Source: CAD feature listing. Evaluate the final solid. Frame: model axes, mm. Round coordinates to 2 decimals unless told otherwise and drop trailing zeros. Order: outer loops, then holes, each group sorted by start corner. A loop starts at its lowest first (then second) coordinate and runs counter-clockwise, first axis right, second up. Notation, with made-up numbers: (-33, 56) - (-21, 56) arc R27 cw to (-21, 95) - close; hole circle Ø2 at (61.5, 56.5). An arc over 180 degrees is marked (long way). Use one line per item in the form item = value. Start each with the question number.
Q1. Cut plane C-C, the plane z = 1.45. Give the number of separate pieces and of enclosed holes in the cut face, and give its area (3 significant figures).
Q2. Cut plane B-B, the plane x = 21. Return the cut outline in (y, z), and give its area (3 significant figures).
Q3. Ray query, line 1 (X direction, y = 41, z = 0.35); line 2 (Y direction, x = 22, z = 0.55); line 3 (Y direction, x = 17, z = 2.55). Return the intervals inside material, ascending. Write a range as [from, to].
Q4. Draft query along X for faces 1 (the flat face through (80.008, 41, 1)), 2 (the flat face through (33, 43, 0)), 3 (the flat face through (59.008, 67, 2)). Return one class per face: released by +X, released by -X, zero draft, split by the parting line, or undercut.
Q5. Cut plane A-A, the plane y = 92.5. Return the cut outline in (x, z), and give its area (3 significant figures).
from build123d import *

# Parameters (mm, degrees)
ESQUISSE1_W             = 120
ESQUISSE1_H             = 140
BOSS_EXTRU_1_DEPTH      = 3
ESQUISSE3_R             = 5
ESQUISSE3_W             = 3
ESQUISSE3_H             = 10
ENL_V_MAT_EXTRU_1_DEPTH = 138.692369665


with BuildPart() as part:
    # Esquisse1 → Boss.-Extru.1 (new body)
    with BuildSketch(Plane.XY):
        with Locations((20.007954742, 42.021943574)):
            Rectangle(ESQUISSE1_W, ESQUISSE1_H)
    extrude(amount=BOSS_EXTRU_1_DEPTH)

    # Esquisse3 → Enlèv. mat.-Extru.1 (cut, through all)
    with BuildSketch(Plane.XY.offset(3)):
        with Locations((20.007954742, 47.021943574)):
            Circle(ESQUISSE3_R)
        with Locations((-20.492045258, 67.021943574)):
            Rectangle(ESQUISSE3_W, ESQUISSE3_H)
        with Locations((-20.492045258, 92.021943574)):
            Rectangle(ESQUISSE3_W, ESQUISSE3_H)
        with Locations((-20.492045258, -7.978056426)):
            Rectangle(ESQUISSE3_W, ESQUISSE3_H)
        with Locations((-20.492045258, 42.021943574)):
            Rectangle(ESQUISSE3_W, ESQUISSE3_H)
        with Locations((-20.492045258, 17.021943574)):
            Rectangle(ESQUISSE3_W, ESQUISSE3_H)
        with Locations((60.507954742, -7.978056426)):
            Rectangle(ESQUISSE3_W, ESQUISSE3_H)
        with Locations((60.507954742, 17.021943574)):
            Rectangle(ESQUISSE3_W, ESQUISSE3_H)
        with Locations((60.507954742, 42.021943574)):
            Rectangle(ESQUISSE3_W, ESQUISSE3_H)
        with Locations((60.507954742, 67.021943574)):
            Rectangle(ESQUISSE3_W, ESQUISSE3_H)
        with Locations((60.507954742, 92.021943574)):
            Rectangle(ESQUISSE3_W, ESQUISSE3_H)
    extrude(amount=-ENL_V_MAT_EXTRU_1_DEPTH, mode=Mode.SUBTRACT)


solid = part.part
Completed:
q1.separate_pieces = 1
q1.enclosed_holes = 11
q1.area = 16,400 mm2
q2.outline = (-27.98, 0) - (42.12, 0) - (42.12, 3) - (-27.98, 3) - close; (51.92, 0) - (112.02, 0) - (112.02, 3) - (51.92, 3) - close
q2.area = 391 mm2
q3.line_1 = [-39.99, -21.99], [-18.99, 59.01], [62.01, 80.01]
q3.line_2 = [-27.98, 42.44], [51.61, 112.02]
q3.line_3 = [-27.98, 43.03], [51.02, 112.02]
q4.face_1 = released by +X
q4.face_2 = zero draft
q4.face_3 = undercut
q5.outline = (-39.99, 0) - (-21.99, 0) - (-21.99, 3) - (-39.99, 3) - close; (-18.99, 0) - (59.01, 0) - (59.01, 3) - (-18.99, 3) - close; (62.01, 0) - (80.01, 0) - (80.01, 3) - (62.01, 3) - close
q5.area = 342 mm2
